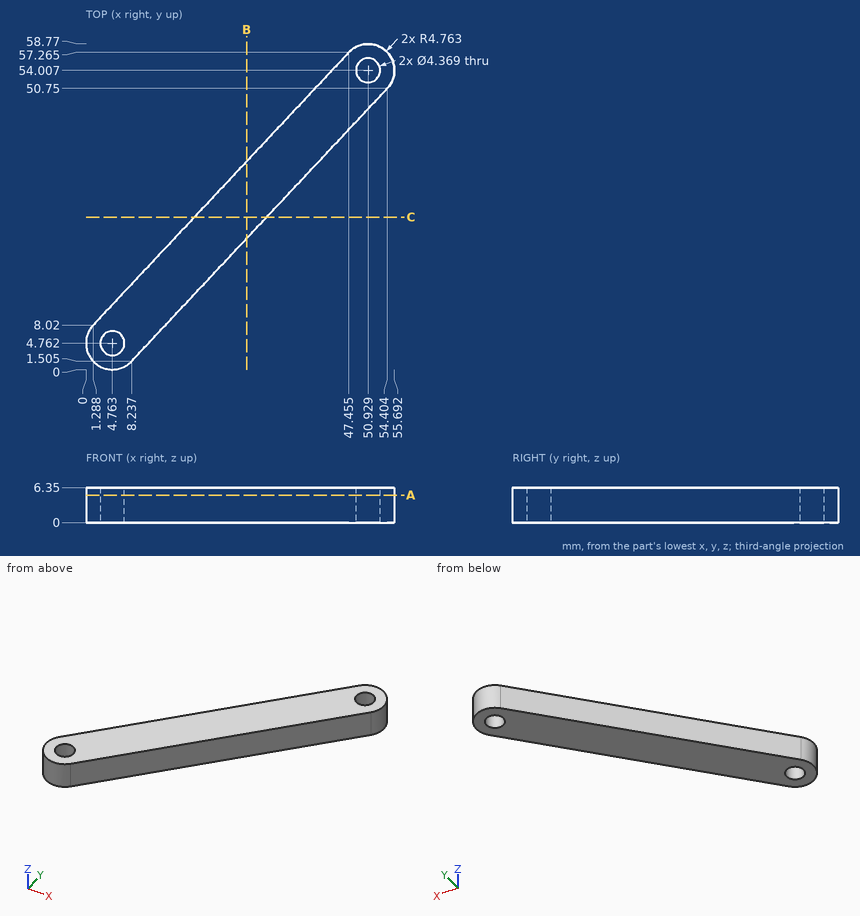
Geometry check sheet. Reference: drawing and pictorial views, mm from the part's lowest x, y, z. Coordinates: 2 decimals unless noted, no trailing zeros. Order: outer loops, then holes, each group sorted by start corner. A loop starts at its lowest first (then second) coordinate and runs counter-clockwise, first axis right, second up. Notation, with made-up numbers: M 54,46.25 L 107,46.25 A29 cw 107,68.25 Z; hole C 10.5,56.25 d7. An arc over 180 degrees is marked long. Return JSON: item names as keys, results as strings.
1) Cross-section at C-C, the plane y = 27.5. Record the boundary of the cut face in (x, z), and give its area (3 significant figures).
Answer list:
{"outline": "M 19.55,0 L 32.61,0 L 32.61,6.35 L 19.55,6.35 Z", "area": "82.9 mm2"}
2) Thickness scan on L1, parallel to X at y = 55, z = 6 (1 decimal); L2, parallel to X at y = 13.5, z = 5.25 (1 decimal); L3, parallel to X at y = 49, z = 3.5 (1 decimal). Record the ranges inside material, lowest first. Write a range as [from, to].
Answer list:
{"L1": "[45.3, 49], [52.9, 55.6]", "L2": "[6.4, 19.5]", "L3": "[39.7, 52.8]"}
3) Cross-section at B-B, the plane x = 29. Record the boundary of the cut face in (y, z).
Answer list:
{"outline": "M 23.65,0 L 37.58,0 L 37.58,6.35 L 23.65,6.35 Z"}
4) Cross-section at A-A, the plane z = 5. Count the separate pieces of the cut face and the enclosed holes in it, and give its area (3 significant figures).
Answer list:
{"separate pieces": "1", "enclosed holes": "2", "area": "684 mm2"}
5) Gauge pin test, flat ends, axial feed: pin 1 (1.5 mm diameter, centred on x = 45, z = 5.5, fed in from +Y) (1 decimal); pin 2 (5.5 mm diameter, centred on x = 4.76, y = 4.76, fed in from -Z); pin 3 (1 mm diameter, centred on x = 9.5, z = 5, fed in from +Y). Record the tip position at first contact, or that the pin passes through.
Answer list:
{"pin 1": "y = 55.4", "pin 2": "z = 0", "pin 3": "y = 17.31"}
